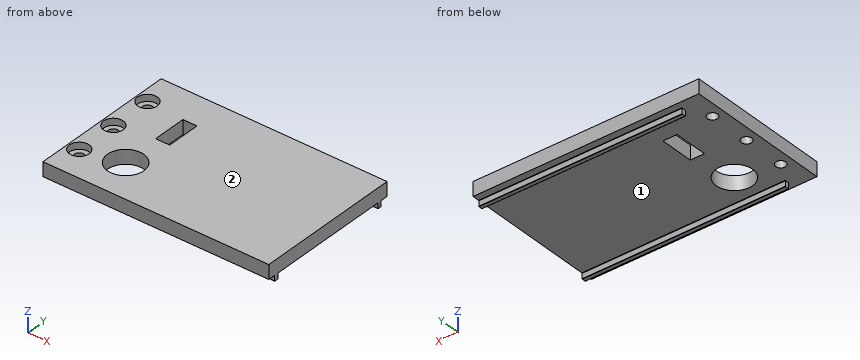
```python
from build123d import *

# Parameters (mm, degrees)
ESQUISSE1_W                                        = 80
ESQUISSE1_H                                        = 52
BOSS_EXTRU_1_DEPTH                                 = 5
ESQUISSE2_R                                        = 6.447859464
ENL_V_MAT_EXTRU_1_DEPTH                            = 5
CHAMBRAGE_POUR_VIS_T_TE_RONDE_BOMB_E_M_D           = 3.6
CHAMBRAGE_POUR_VIS_T_TE_RONDE_BOMB_E_M_CBORE_D     = 7
CHAMBRAGE_POUR_VIS_T_TE_RONDE_BOMB_E_M_CBORE_DEPTH = 2.4
ESQUISSE5_W                                        = 72
ESQUISSE5_H                                        = 1.45
BOSS_EXTRU_2_DEPTH                                 = 2
CONG_1_R                                           = 0.1
ESQUISSE6_W                                        = 5
ESQUISSE6_H                                        = 12
ENL_V_MAT_EXTRU_2_DEPTH                            = 99.420026836


with BuildPart() as part:
    # Esquisse1 → Boss.-Extru.1 (new body)
    with BuildSketch(Plane.XY.offset(16.98011664)):
        with Locations((-44.444303066, 24.066569306)):
            Rectangle(ESQUISSE1_W, ESQUISSE1_H)
    extrude(amount=BOSS_EXTRU_1_DEPTH)

    # Esquisse2 → Enlèv. mat.-Extru.1 (cut)
    with BuildSketch(Plane.XY.offset(21.98011664)):
        with Locations((-66.444303066, 12.061734253)):
            Circle(ESQUISSE2_R)
    extrude(amount=-ENL_V_MAT_EXTRU_1_DEPTH, mode=Mode.SUBTRACT)

    # Chambrage pour vis à tête ronde bombée M34 (through all)
    with Locations(Plane.XY.offset(21.98011664)):
        with Locations((-80.444303066, 9.066569306), (-80.444303066, 24.066569306), (-80.444303066, 39.066569306)):
            CounterBoreHole(CHAMBRAGE_POUR_VIS_T_TE_RONDE_BOMB_E_M_D / 2, CHAMBRAGE_POUR_VIS_T_TE_RONDE_BOMB_E_M_CBORE_D / 2, CHAMBRAGE_POUR_VIS_T_TE_RONDE_BOMB_E_M_CBORE_DEPTH)

    # Esquisse5 → Boss.-Extru.2 (add)
    with BuildSketch(Plane(origin=(0, 0, 16.98011664), x_dir=(-1, 0, 0), z_dir=(0, 0, -1))):
        with Locations((40.444303066, 1.341569306)):
            Rectangle(ESQUISSE5_W, ESQUISSE5_H)
        with Locations((40.444303066, 46.791569306)):
            Rectangle(ESQUISSE5_W, ESQUISSE5_H)
    extrude(amount=BOSS_EXTRU_2_DEPTH)

    # Congé1
    cong_1_edges = [part.edges().sort_by_distance(p)[0] for p in [
        (-40.444303066, 0.616569306, 16.98011664),
        (-40.444303066, 2.066569306, 16.98011664),
        (-40.444303066, 0.616569306, 14.98011664),
        (-40.444303066, 2.066569306, 14.98011664),
        (-40.444303066, 46.066569306, 16.98011664),
        (-40.444303066, 47.516569306, 16.98011664),
        (-40.444303066, 46.066569306, 14.98011664),
        (-40.444303066, 47.516569306, 14.98011664),
    ]]
    fillet(cong_1_edges, radius=CONG_1_R)

    # Esquisse6 → Enlèv. mat.-Extru.2 (cut, through all)
    with BuildSketch(Plane.XY.offset(21.98011664)):
        with Locations((-64.788459284, 32.318430869)):
            Rectangle(ESQUISSE6_W, ESQUISSE6_H)
    extrude(amount=-ENL_V_MAT_EXTRU_2_DEPTH, mode=Mode.SUBTRACT)


solid = part.part
```
Could you check a few things on this model? Use its own coordinates, in mm. Face numbers are marked on the shaded views. Round coordinates to 2 decimals unless told otherwise and drop trailing zeros. Loops run counter-clockwise (first coordinate to the right, second up) from the corner with the lowest first, then second, coordinate; pieces in that order, holes last. Notation, with made-up numbers: (23, 84.5) -> (81, 84.5) arc R15 cw to (81, 109.5) -> close; hole circle Ø9 at (-28.75, 80.25). An arc over 180 degrees is marked (long way). Put each result on its own line as item: value.
Q1. Please list where these lines run through material, in increasing order: line 1 (X direction, y = 32, z = 19.5); line 2 (Y direction, x = -67, z = 18.5); line 3 (Y direction, x = -11.5, z = 15.5). Write a range as from..to.
Checks:
line 1: -84.44..-67.29, -62.29..-4.44
line 2: -1.93..5.64, 18.49..26.32, 38.32..50.07
line 3: 0.62..2.07, 46.07..47.52
Q2. Thinking about a two-plate mould opening in Y: for the marked faces 1 and 2, which applies, pulls with the +Y half, pulls with the -Y half, needs draft (parallel to the pull), parting line crosses it, or undercut?
Checks:
face 1: undercut
face 2: needs draft
Q3. I want a section at A-A on y = 29.5. Write out the boundary of the cut face in (x, z).
Checks:
outline: (-84.44, 16.98) -> (-67.29, 16.98) -> (-67.29, 21.98) -> (-84.44, 21.98) -> close; (-62.29, 16.98) -> (-4.44, 16.98) -> (-4.44, 21.98) -> (-62.29, 21.98) -> close
Q4. For pin 1 Ø11 at (x, y) = (-80.44, 39.07) entering from +Z; pin 2 Ø6 at (x, y) = (-80.44, 24.07) entering from +Z; pin 3 Ø3 at (x, y) = (-13.5, 30.5) entering from -Z; pin 4 Ø2 at (x, z) = (-53, 15.5) entering from +Y, each with a flat end and sliding along its axis, tell me the tip position at first contact or that it passes through.
Checks:
pin 1: z = 21.98
pin 2: z = 19.58
pin 3: z = 16.98
pin 4: y = 47.52
Q5. I want a section at D-D on z = 20.5. Write out the boundary of the cut face in (x, y), and give its area (3 significant figures).
Checks:
outline: (-84.44, -1.93) -> (-4.44, -1.93) -> (-4.44, 50.07) -> (-84.44, 50.07) -> close; hole circle Ø7 at (-80.44, 9.07); hole circle Ø7 at (-80.44, 24.07); hole circle Ø7 at (-80.44, 39.07); hole circle Ø12.9 at (-66.44, 12.06); hole (-67.29, 26.32) -> (-62.29, 26.32) -> (-62.29, 38.32) -> (-67.29, 38.32) -> close
area: 3,850 mm2
Q6. I want a section at B-B on z = 16. Write out the boundary of the cut face in (x, y), and give its area (3 significant figures).
Checks:
outline: (-76.44, 0.62) -> (-4.44, 0.62) -> (-4.44, 2.07) -> (-76.44, 2.07) -> close; (-76.44, 46.07) -> (-4.44, 46.07) -> (-4.44, 47.52) -> (-76.44, 47.52) -> close
area: 209 mm2
Q7. I want a section at C-C on x = -72. Write out the boundary of the cut face in (y, z).
Checks:
outline: (-1.93, 16.98) -> (0.52, 16.98) arc R0.1 cw to (0.62, 16.88) -> (0.62, 15.08) arc R0.1 ccw to (0.72, 14.98) -> (1.97, 14.98) arc R0.1 ccw to (2.07, 15.08) -> (2.07, 16.88) arc R0.1 cw to (2.17, 16.98) -> (8.79, 16.98) -> (8.79, 21.98) -> (-1.93, 21.98) -> close; (15.33, 16.98) -> (45.97, 16.98) arc R0.1 cw to (46.07, 16.88) -> (46.07, 15.08) arc R0.1 ccw to (46.17, 14.98) -> (47.42, 14.98) arc R0.1 ccw to (47.52, 15.08) -> (47.52, 16.88) arc R0.1 cw to (47.62, 16.98) -> (50.07, 16.98) -> (50.07, 21.98) -> (15.33, 21.98) -> close
